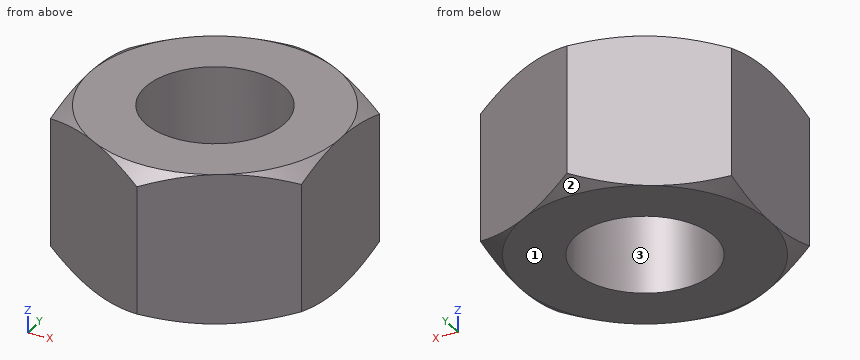
```python
from build123d import *

# Parameters (mm, degrees)
BASENUTSKE_R  = 3.96875
BASENUT_DEPTH = 8.5598


with BuildPart() as part:
    # BaseNutSke → BaseNut (new body)
    with BuildSketch(Plane.XY):
        Polygon((7.1374, 4.120779811), (7.1374, -4.120779811), (0, -8.241559623), (-7.1374, -4.120779811), (-7.1374, 4.120779811), (0, 8.241559623), align=None)
        Circle(BASENUTSKE_R, mode=Mode.SUBTRACT)
    extrude(amount=-BASENUT_DEPTH)

    # Sketch3 → Double-Chamfer (revolve, cut)
    with BuildSketch(Plane(origin=(0, 0, 0), x_dir=(0, 0, -1), z_dir=(1, 0, 0))):
        Polygon((8.5598, 7.1374), (7.9248, 8.241559623), (7.9248, 20.941559623), (21.2598, 20.941559623), (21.2598, 7.1374), align=None)
        Polygon((0.635, 20.941559623), (-12.7, 20.941559623), (-12.7, 7.1374), (0, 7.1374), (0.635, 8.241559623), align=None)
    revolve(axis=Axis((0, 0, 0), (0, 0, -1)), mode=Mode.SUBTRACT)

    # Sketch5 → EndChamfer (revolve, cut)
    with BuildSketch(Plane(origin=(0, 0, 0), x_dir=(0, 0, -1), z_dir=(1, 0, 0))):
        Polygon((8.5344, 3.175), (8.055086934, 2.49047), (8.5852, 2.49047), (8.5852, 3.175), align=None)
        Polygon((-0.0508, 3.175), (0, 3.175), (0.479313066, 2.49047), (-0.0508, 2.49047), align=None)
    revolve(axis=Axis((0, 0, -25.037505729), (0, 0, -1)), mode=Mode.SUBTRACT)


solid = part.part
```
Verification items for the finished model (mm, model axes). Face numbers are marked on the shaded views. Coordinates: 2 decimals unless noted, no trailing zeros. Write each loop counter-clockwise with the first axis right and the second up, starting at its lowest first coordinate (ties: lowest second). Pieces come first, ordered by that corner, then holes. Notation, with made-up numbers: M 63.5,-38 L 86.5,-38 A21 ccw 86.5,-5 Z; hole C -4,-14 d6. An arc over 180 degrees is marked long. Answer as a JSON object with one key per item and string values. Group by question number.
(1) Material ranges on line 1 (Y direction, x = -2.5, z = -1.75); line 2 (X direction, y = -3, z = -4.5); line 3 (Y direction, x = -2, z = -0.5), recorded low to high.
(2) Release check for a two-part mould opening along Y. For the marked faces 1, 2 and 3 record: +Y half, -Y half, draft (parallel to the pull), parting line (faces both ways), or undercut.
(3) Cross-section at A-A, the plane z = -1.75. Record the cut outline in (x, y).
Reply:
{
 "1": {"line 1": "-6.8 to -3.08, 3.08 to 6.8", "line 2": "-7.14 to -2.6, 2.6 to 7.14", "line 3": "-7.09 to -3.43, 3.43 to 7.09"},
 "2": {"face 1": "draft", "face 2": "+Y half", "face 3": "undercut"},
 "3": {"outline": "M -7.14,-4.12 L 0,-8.24 L 7.14,-4.12 L 7.14,4.12 L 0,8.24 L -7.14,4.12 Z; hole C 0,0 d7.94"}
}
